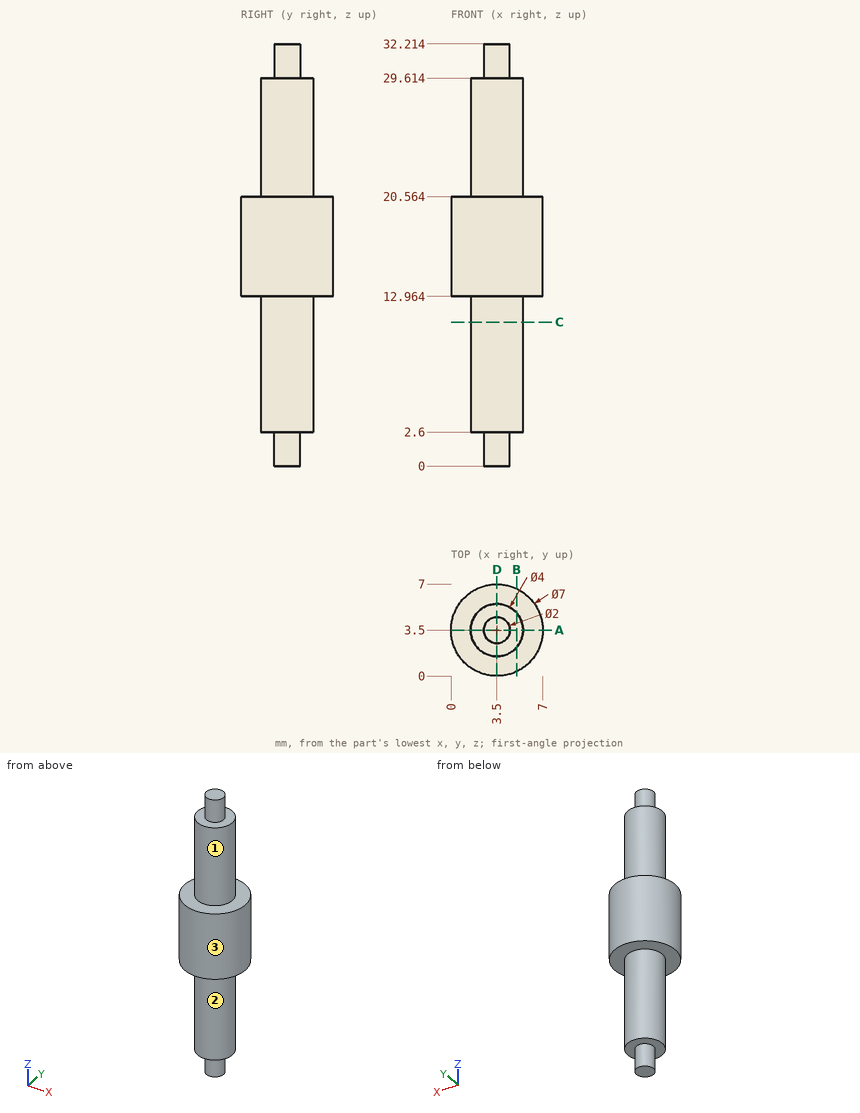
Verification items for this drawing (mm, ordinates from the low corner). A direction names the side the tool comes from. Give positions to 0.01 mm unless a question says otherwise; leave off trailing zeros. Loops run counter-clockwise (first coordinate to the right, second up) from the corner with the lowest first, then second, coordinate; pieces in that order, holes last. Notation, with made-up numbers: M 0.5,48 L 28.5,48 A24 ccw 28.5,79 Z; hole C -5,87 d2. An arc over 180 degrees is marked long. Answer as a JSON object with one key per item and string values. Group by question number.
Item 1: Sectioned sample at C-C on z = 11. Record the boundary of the cut face in (x, y), plus the area to 3 significant figures.
Item 2: Material ranges on L1, parallel to Z at x = 4.75, y = 4; L2, parallel to Z at x = 1.5, y = 6; L3, parallel to X at y = 5, z = 29 (1 decimal), recorded low to high.
Item 3: Gauge pin test, flat ends, axial feed: pin 1 (2 mm diameter, centred on x = 6, y = 6.5, fed in from +Z); pin 2 (1.5 mm diameter, centred on x = 2, y = 5.5, fed in from +Z); pin 3 (1 mm diameter, centred on x = 5.5, z = 16, fed in from -Y). Record the tip position at first contact, or that the pin passes through.
Item 4: Sectioned sample at B-B on x = 5. Record the boundary of the cut face in (y, z).
Item 5: Sectioned sample at A-A on y = 3.5. Record the boundary of the cut face in (x, z), plus the area to 3 significant figures.
Item 6: Access from +Z, -Z, +X, -X, +Y, -Y to the whole of each face (thin tool, end or side, straight path). Record for the marked faces 1, 2 and 3.
Findings below:
{
 "1": {"outline": "C 3.5,3.5 d4", "area": "12.6 mm2"},
 "2": {"L1": "2.6 to 29.61", "L2": "12.96 to 20.56", "L3": "2.2 to 4.8"},
 "3": {"pin 1": "z = 20.56", "pin 2": "z = 29.61", "pin 3": "y = 0.34"},
 "4": {"outline": "M 0.34,12.96 L 2.18,12.96 L 2.18,2.6 L 4.82,2.6 L 4.82,12.96 L 6.66,12.96 L 6.66,20.56 L 4.82,20.56 L 4.82,29.61 L 2.18,29.61 L 2.18,20.56 L 0.34,20.56 Z"},
 "5": {"outline": "M 0,12.96 L 1.5,12.96 L 1.5,2.6 L 2.5,2.6 L 2.5,0 L 4.5,0 L 4.5,2.6 L 5.5,2.6 L 5.5,12.96 L 7,12.96 L 7,20.56 L 5.5,20.56 L 5.5,29.61 L 4.5,29.61 L 4.5,32.21 L 2.5,32.21 L 2.5,29.61 L 1.5,29.61 L 1.5,20.56 L 0,20.56 Z", "area": "141 mm2"},
 "6": {"face 1": "+Z", "face 2": "-Z", "face 3": "+Z, -Z"}
}
